```python
from build123d import *

# Parameters (mm, degrees)
SKETCH1_R             = 14
BOSS_EXTRUDE1_DEPTH   = 14.5
SKETCH2_R             = 8
BOSS_EXTRUDE2_DEPTH   = 5.5
SKETCH3_W             = 5.27
SKETCH3_H             = 10.5
SKETCH4_R             = 4
CUT_EXTRUDE1_DEPTH    = 29.142494559
SKETCH5_W             = 3
SKETCH5_H             = 2.8
CUT_EXTRUDE2_DEPTH    = 29.142494559
M4_TAPPED_HOLE1_D     = 3.3
M4_TAPPED_HOLE1_DEPTH = 5
M4_TAPPED_HOLE1_TIP   = 0.991420021


with BuildPart() as part:
    # Sketch1 → Boss-Extrude1 (new body)
    with BuildSketch(Plane(origin=(0, 0, 0), x_dir=(1, 0, 0), z_dir=(0, 1, 0))):
        with Locations(Location((0, 0, 0), (0, 0, 90))):
            Circle(SKETCH1_R)
    extrude(amount=BOSS_EXTRUDE1_DEPTH)

    # Sketch2 → Boss-Extrude2 (add)
    with BuildSketch(Plane(origin=(0, 14.5, 0), x_dir=(1, 0, 0), z_dir=(0, 1, 0))):
        with Locations(Location((0, 0, 0), (0, 0, 270))):
            Circle(SKETCH2_R)
    extrude(amount=BOSS_EXTRUDE2_DEPTH)

    # Sketch3 → Cut-Revolve1 (revolve, cut)
    with BuildSketch(Plane(origin=(0, 0, 0), x_dir=(0, 0, -1), z_dir=(1, 0, 0)), mode=Mode.PRIVATE) as cut_revolve1_sk:
        with Locations((-14, 7.25)):
            Rectangle(SKETCH3_W, SKETCH3_H)
    revolve(cut_revolve1_sk.sketch.rotate(Axis((0, 14.5, 0), (0, -1, 0)), 180), axis=Axis((0, 14.5, 0), (0, -1, 0)), mode=Mode.SUBTRACT)

    # Sketch4 → Cut-Extrude1 (cut, through all)
    with BuildSketch(Plane(origin=(0, 20, 0), x_dir=(1, 0, 0), z_dir=(0, 1, 0))):
        with Locations(Location((0, 0, 0), (0, 0, 270))):
            Circle(SKETCH4_R)
    extrude(amount=-CUT_EXTRUDE1_DEPTH, mode=Mode.SUBTRACT)

    # Sketch5 → Cut-Extrude2 (cut, through all)
    with BuildSketch(Plane(origin=(0, 20, 0), x_dir=(1, 0, 0), z_dir=(0, 1, 0))):
        with Locations((0, 4)):
            Rectangle(SKETCH5_W, SKETCH5_H)
    extrude(amount=-CUT_EXTRUDE2_DEPTH, mode=Mode.SUBTRACT)

    # M4 Tapped Hole1
    with Locations(Plane(origin=(0, 17.25, 8), x_dir=(1, 0, 0), z_dir=(0, 0, 1))):
        with Locations((0, 0)):
            Hole(M4_TAPPED_HOLE1_D / 2, depth=M4_TAPPED_HOLE1_DEPTH)
            with Locations((0, 0, -(M4_TAPPED_HOLE1_DEPTH + M4_TAPPED_HOLE1_TIP / 2))):  # 118° drill point
                Cone(0, M4_TAPPED_HOLE1_D / 2, M4_TAPPED_HOLE1_TIP, mode=Mode.SUBTRACT)


solid = part.part
```
Design review of the part built by this model. Coordinates are the model's own, in mm. A direction names the side the tool comes from. Coordinates: 2 decimals unless noted, no trailing zeros. Write each loop counter-clockwise with the first axis right and the second up, starting at its lowest first coordinate (ties: lowest second). Pieces come first, ordered by that corner, then holes. Notation, with made-up numbers: M 81.25,-35.75 L 128.25,-35.75 A19 cw 128.25,-16.75 Z; hole C -25.75,3 d10. An arc over 180 degrees is marked long. Answer as a JSON object with one key per item and string values.
Item 1: Add section C-C, the plane y = 7.25. Give the boundary of the cut face in (x, z) (3 decimals), and give its area (3 significant figures).
Outcome:
{"outline": "C 0,0 d22.73; hole M -1.5,-5.4 L 1.5,-5.4 L 1.5,-3.708 A4 ccw long -1.5,-3.708 Z", "area": "351 mm²"}
Item 2: Draft analysis for pull direction X (two halves, no side actions). For faces 1 (the flat face through (0, 10, -5.4)), 2 (the flat face through (-2, 20, -4)), 3 (the cylindrical face through (13.67, 13.49, 3.03)), state which applies: pulls with the +X half, pulls with the -X half, needs draft (parallel to the pull), parting line crosses it, or undercut.
Outcome:
{"face 1": "undercut", "face 2": "needs draft", "face 3": "parting line crosses it"}
Item 3: Add section B-B, the plane z = 0. Give the boundary of the cut face in (x, y) (3 decimals).
Outcome:
{"outline": "M -14,0 L -4,0 L -4,20 L -8,20 L -8,14.5 L -14,14.5 L -14,12.5 L -11.365,12.5 L -11.365,2 L -14,2 Z; M 4,0 L 14,0 L 14,2 L 11.365,2 L 11.365,12.5 L 14,12.5 L 14,14.5 L 8,14.5 L 8,20 L 4,20 Z"}
Item 4: Wall thickness on probe 1 along Y at (x, z) = (11.75, 2.5); probe 2 along X at (y, z) = (6, 0) (3 decimals); probe 3 along X at (y, z) = (14.25, 0): over which ranges is each line inside the solid? List them lowest first.
Outcome:
{"probe 1": "0 to 2, 12.5 to 14.5", "probe 2": "-11.365 to -4, 4 to 11.365", "probe 3": "-14 to -4, 4 to 14"}
Item 5: Add section D-D, the plane x = -3.25. Give the boundary of the cut face in (y, z).
Outcome:
{"outline": "M 0,-13.62 L 2,-13.62 L 2,-10.89 L 12.5,-10.89 L 12.5,-13.62 L 14.5,-13.62 L 14.5,-7.31 L 20,-7.31 L 20,-2.33 L 0,-2.33 Z; M 0,2.33 L 20,2.33 L 20,7.31 L 14.5,7.31 L 14.5,13.62 L 12.5,13.62 L 12.5,10.89 L 2,10.89 L 2,13.62 L 0,13.62 Z"}
Item 6: Add section A-A, the plane x = 0. Give the boundary of the cut face in (y, z) (3 decimals), and give its area (3 significant figures).
Outcome:
{"outline": "M 0,-14 L 2,-14 L 2,-11.365 L 12.5,-11.365 L 12.5,-14 L 14.5,-14 L 14.5,-8 L 20,-8 L 20,-5.4 L 0,-5.4 Z; M 0,4 L 15.6,4 L 15.6,8 L 14.5,8 L 14.5,14 L 12.5,14 L 12.5,11.365 L 2,11.365 L 2,14 L 0,14 Z; M 18.9,4 L 20,4 L 20,8 L 18.9,8 Z", "area": "237 mm²"}
Item 7: Machinability: for faces 4 (the cylindrical face through (-7.81, 17.21, -1.73)), 5 (the flat face through (11.5, 2, 1.1)), 6 (the cylindrical face through (1.65, 17.32, 5.79)), which of the approach directions +Z, -Z, +X, -X, +Y, -Y give a long, thin tool a straight path to every point of the face, cutting with its end or side? Answer none if there is none.
Outcome:
{"face 4": "+Y", "face 5": "none", "face 6": "+Z"}
Item 8: Insertion check: pin 1 Ø1.5 at (x, y) = (10, 2) entering from +Z; pin 2 Ø1.5 at (x, y) = (6.5, 12) entering from +Z; pin 3 Ø6 at (x, z) = (3, 6.5) entering from -Y; pin 4 Ø0.5 at (y, z) = (10, -4.5) entering from -X. Each pin has a flat end and moves straight along its axis. Give the tip position at first contact, or say it passes through.
Outcome:
{"pin 1": "z = 10.51", "pin 2": "z = 12.68", "pin 3": "y = 0", "pin 4": "x = -10.54"}
